from build123d import *

# Parameters (mm, degrees)
SKETCH_1_W             = 100
SKETCH_1_H             = 100
EXTRUDE_1_DEPTH        = 1960
SKETCH_2_W             = 88
SKETCH_2_H             = 88
CUT_EXTRUDE_1_DEPTH    = 1966.095417531
SKETCH_3_R             = 13
CUT_EXTRUDE_2_DEPTH    = 1965.521315741
PATTERN_LINEAR_1_COUNT = 4
PATTERN_LINEAR_1_PITCH = 80
SKETCH_4_R             = 13
CUT_EXTRUDE_3_DEPTH    = 1965.521315741
PATTERN_LINEAR_2_COUNT = 4
PATTERN_LINEAR_2_PITCH = 80


with BuildPart() as part:
    # 草图1 → 凸台-拉伸1 (new body)
    with BuildSketch(Plane.XY):
        with Locations((50, 50)):
            Rectangle(SKETCH_1_W, SKETCH_1_H)
    extrude(amount=EXTRUDE_1_DEPTH)

    # 草图2 → 切除-拉伸1 (cut, through all)
    with BuildSketch(Plane.XY.offset(1960)):
        with Locations((56, 56)):
            Rectangle(SKETCH_2_W, SKETCH_2_H)
    extrude(amount=-CUT_EXTRUDE_1_DEPTH, mode=Mode.SUBTRACT)

    # 草图3 → 切除-拉伸2 (cut, through all)
    with BuildSketch(Plane(origin=(12, 0, 0), x_dir=(0, 0, -1), z_dir=(1, 0, 0))):
        with Locations(Location((-1910, 60, 0), (0, 0, 90))):
            Circle(SKETCH_3_R)
    cut_extrude_2 = extrude(amount=-CUT_EXTRUDE_2_DEPTH, mode=Mode.SUBTRACT)

    # 阵列(线性)1: 切除-拉伸2 ×4
    with Locations(*[(0, 0, -i * PATTERN_LINEAR_1_PITCH) for i in range(1, PATTERN_LINEAR_1_COUNT)]):
        add(cut_extrude_2, mode=Mode.SUBTRACT)

    # 草图4 → 切除-拉伸3 (cut, through all)
    with BuildSketch(Plane(origin=(12, 0, 0), x_dir=(0, 0, -1), z_dir=(1, 0, 0))):
        with Locations(Location((-170, 60, 0), (0, 0, 90))):
            Circle(SKETCH_4_R)
    cut_extrude_3 = extrude(amount=-CUT_EXTRUDE_3_DEPTH, mode=Mode.SUBTRACT)

    # 阵列(线性)2: 切除-拉伸3 ×4
    with Locations(*[(0, 0, i * PATTERN_LINEAR_2_PITCH) for i in range(1, PATTERN_LINEAR_2_COUNT)]):
        add(cut_extrude_3, mode=Mode.SUBTRACT)


solid = part.part
Check sheet for the modelled part. Datum: model origin and axes. Units: mm. A direction names the side the tool comes from. Round coordinates to 2 decimals unless told otherwise and drop trailing zeros. Order: outer loops, then holes, each group sorted by start corner. A loop starts at its lowest first (then second) coordinate and runs counter-clockwise, first axis right, second up.
(1) Go/stop test with flat-tipped pins: P1, Ø4, axis at x = 50, z = 429, coming from the -Y side; P2, Ø21, axis at y = 60, z = 250, coming from the -X side. Record where each tip stops, or that it passes through.
(2) Cross-section at B-B, the plane z = 1483.5. Enter the section's corners in (x, y).
(3) Cross-section at A-A, the plane x = 65. Enter the section's corners in (y, z), and give its area (3 significant figures).
(4) Access from +Z, -Z, +X, -X, +Y, -Y to the whole of each face (thin tool, end or side, straight path). Record for faces 1 (the flat face through (12, 55, 994)), 2 (the flat face through (28, 9, 0)).
(5) Scan line: probe 1 along Y at (x, z) = (26, 809). Record every from-to range of solid material in increasing order.
Check sheet entries:
1. P1: stops at y = 0
1. P2: passes through
2. outline: (0, 0) - (100, 0) - (100, 12) - (12, 12) - (12, 100) - (0, 100) - close
3. outline: (0, 0) - (12, 0) - (12, 1960) - (0, 1960) - close
3. area: 23,500 mm2
4. face 1: +Z, -Z, +X, +Y
4. face 2: -Z, +X, -X, +Y, -Y
5. probe 1: y = 0 to 12
